```python
from build123d import *

# Parameters (mm, degrees)
F0_W     = 64.0385448933
F0_H     = 53.5832680762
F1_DEPTH = 25.4
F2_T     = -2.54
F3_W     = 46.9654425979
F3_H     = 35.9974689782
F4_DEPTH = 76.2
F5_W     = 46.9654425979
F5_H     = 35.9974689782
F6_DEPTH = 25.4


with BuildPart() as f1:
    # F0 (on Top) → F1 (new body)
    with BuildSketch(Plane.XY):
        with Locations((14.1581892967, 1.3069082052)):
            Rectangle(F0_W, F0_H)
    extrude(amount=F1_DEPTH)

    # F2
    f2_openings = [f1.faces().sort_by_distance(p)[0] for p in [
        (14.158189, 1.306908, 25.4),
    ]]
    offset(amount=F2_T, openings=f2_openings)

    # F3 (on Top) → F4 (join)
    with BuildSketch(Plane.XY):
        with Locations((14.3955796957, 0.8823070675)):
            Rectangle(F3_W, F3_H)
    extrude(amount=F4_DEPTH)

    # F5 (on face) → F6 (join)
    with BuildSketch(Plane.XY.offset(76.2)):
        with Locations((14.3955796957, 0.8823070675)):
            Rectangle(F5_W, F5_H)
    extrude(amount=F6_DEPTH)


solid = f1.part
```
Could you check a few things on this model? Use its own coordinates, in mm. A direction names the side the tool comes from. Round coordinates to 2 decimals unless told otherwise and drop trailing zeros. Loops run counter-clockwise (first coordinate to the right, second up) from the corner with the lowest first, then second, coordinate; pieces in that order, holes last. Notation, with made-up numbers: (-38, 85) -> (-13, 85) arc R16 ccw to (-13, 104) -> close; hole circle Ø11 at (1.25, 3.5). An arc over 180 degrees is marked (long way). One line per question, with ' | ' between items.
(1) If we section it at D-D on x = 29: List the corners of the cut face in (y, z) for me.
Model answer:
outline: (-25.48, 0) -> (28.1, 0) -> (28.1, 25.4) -> (25.56, 25.4) -> (25.56, 2.54) -> (18.88, 2.54) -> (18.88, 101.6) -> (-17.12, 101.6) -> (-17.12, 2.54) -> (-22.94, 2.54) -> (-22.94, 25.4) -> (-25.48, 25.4) -> close
(2) Thinking about a two-plate mould opening in Y: for faces 1 (the face through (14, -17.116, 51)), 2 (the face through (14, 28.099, 13)), 3 (the face through (46.177, 1, 13)), 4 (the face through (14, -25.485, 13)), which applies, released by +Y, released by -Y, zero draft, split by the parting line, or undercut?
Model answer:
face 1: undercut | face 2: released by +Y | face 3: zero draft | face 4: released by -Y
(3) If we section it at A-A on z = 8: List the corners of the cut face in (x, y) for me, and give its area (3 significant figures).
Model answer:
outline: (-17.86, -25.48) -> (46.18, -25.48) -> (46.18, 28.1) -> (-17.86, 28.1) -> close; (-9.09, -17.12) -> (37.88, -17.12) -> (37.88, 18.88) -> (-9.09, 18.88) -> close; hole (-15.32, -22.94) -> (43.64, -22.94) -> (43.64, 25.56) -> (-15.32, 25.56) -> close | area: 2,260 mm^2
(4) If I drill on probe 1 along X at (y, z) = (-15, 11); probe 2 along X at (y, z) = (22.5, 19); probe 3 along Y at (x, z) = (11, 12), over which ranges is the centre line in solid material (lowest first)?
Model answer:
probe 1: x = -17.86 to -15.32, -9.09 to 37.88, 43.64 to 46.18 | probe 2: x = -17.86 to -15.32, 43.64 to 46.18 | probe 3: y = -25.48 to -22.94, -17.12 to 18.88, 25.56 to 28.1
(5) For faces 5 (the face through (14, 2, 0)), 6 (the face through (14, -22.945, 14)), which set-ups out of +Z, -Z, +X, -X, +Y, -Y let a thin tool reach every point of the face, with its end or its side?
Model answer:
face 5: -Z, +X, -X, +Y, -Y | face 6: +Z
(6) If we section it at B-B on x = 39.5: List the corners of the cut face in (y, z) for me, and give its area (3 significant figures).
Model answer:
outline: (-25.48, 0) -> (28.1, 0) -> (28.1, 25.4) -> (25.56, 25.4) -> (25.56, 2.54) -> (-22.94, 2.54) -> (-22.94, 25.4) -> (-25.48, 25.4) -> close | area: 252 mm^2
(7) If we section it at C-C on y = 21: List the corners of the cut face in (x, z) for me, and give its area (3 significant figures).
Model answer:
outline: (-17.86, 0) -> (46.18, 0) -> (46.18, 25.4) -> (43.64, 25.4) -> (43.64, 2.54) -> (-15.32, 2.54) -> (-15.32, 25.4) -> (-17.86, 25.4) -> close | area: 279 mm^2
(8) For pin 1 Ø1 at (y, z) = (4, 61.5) entering from +X; pin 2 Ø18 at (y, z) = (-0.5, 66.5) entering from -X; pin 3 Ø2 at (x, z) = (35, 59) entering from +Y; pin 4 Ø1 at (x, z) = (-10.5, 36) entering from +Y, each with a flat end and sliding along its axis, tell me the tip position at first contact or that it passes through.
Model answer:
pin 1: stops at x = 37.88 | pin 2: stops at x = -9.09 | pin 3: stops at y = 18.88 | pin 4: passes through
